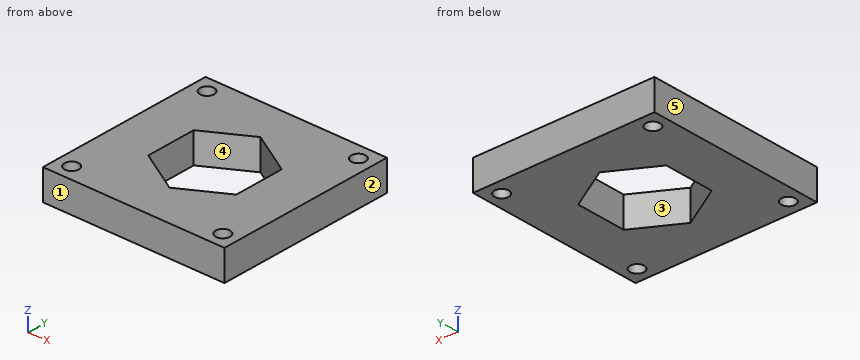
Autodesk Fusion 360 part; units mm, degrees
sketch "Sketch1" plane through (0, 0, 0) normal (0, 0, 1) x (1, 0, 0)
  line L0 (18.48, 10.6694) -> (0, 21.3389)
  line L1 (0, 21.3389) -> (-18.48, 10.6694)
  line L2 (-18.48, 10.6694) -> (-18.48, -10.6694)
  line L3 (-18.48, -10.6694) -> (0, -21.3389)
  line L4 (0, -21.3389) -> (18.48, -10.6694)
  line L5 (18.48, -10.6694) -> (18.48, 10.6694)
  line L6 (38.1, -38.1) -> (-38.1, -38.1)
  line L7 (-38.1, -38.1) -> (-38.1, 38.1)
  line L8 (-38.1, 38.1) -> (38.1, 38.1)
  line L9 (38.1, 38.1) -> (38.1, -38.1)
  line L10 (38.1, -38.1) -> (-38.1, 38.1) construction
  line L11 (-38.1, -38.1) -> (38.1, 38.1) construction
  line L12 (31.75, 31.75) -> (-31.75, 31.75) construction
  line L13 (-31.75, 31.75) -> (-31.75, -31.75) construction
  line L14 (-31.75, -31.75) -> (31.75, -31.75) construction
  line L15 (31.75, -31.75) -> (31.75, 31.75) construction
  line L16 (31.75, 31.75) -> (-31.75, -31.75) construction
  line L17 (-31.75, 31.75) -> (31.75, -31.75) construction
  circle A0 centre (-31.75, 31.75) radius 3
  circle A1 centre (-31.75, -31.75) radius 3
  circle A2 centre (31.75, -31.75) radius 3
  circle A3 centre (31.75, 31.75) radius 3
  dimension "d1" = 18.48
  dimension "d2" = 76.2
  dimension "d3" = 76.2
  dimension "d4" = 63.5
  dimension "d5" = 63.5
  dimension "d6" = 6
  dimension "d8" = 360
extrude "Extrude1" add sketch "Sketch1" along normal blind 12.7
sketch "Sketch2" plane through (0, 0, 12.7) normal (0, 0, 1) x (-1, 0, 0)
  circle A0 centre (31.75, 31.75) radius 3
  circle A1 centre (-31.75, -31.75) radius 3
  line L0 (-18.48, -10.6694) -> (-18.48, 10.6694)
  line L1 (-18.48, 10.6694) -> (0, 21.3389)
  line L2 (0, 21.3389) -> (18.48, 10.6694)
  line L3 (18.48, 10.6694) -> (18.48, -10.6694)
  line L4 (18.48, -10.6694) -> (0, -21.3389)
  line L5 (0, -21.3389) -> (-18.48, -10.6694)
  circle A2 centre (-31.75, 31.75) radius 3
  circle A3 centre (31.75, -31.75) radius 3
  line L6 (-38.1, -38.1) -> (38.1, -38.1)
  line L7 (38.1, -38.1) -> (38.1, 38.1)
  line L8 (38.1, 38.1) -> (-38.1, 38.1)
  line L9 (-38.1, 38.1) -> (-38.1, -38.1)
The listing builds one solid part. Answer for the finished solid, in the listing's coordinates (mm). Face numbers are marked on the shaded views. A direction names the side the tool comes from. Coordinates: 2 decimals unless noted, no trailing zeros. Write each loop counter-clockwise with the first axis right and the second up, starting at its lowest first coordinate (ties: lowest second). Pieces come first, ordered by that corner, then holes. Notation, with made-up numbers: M 17.5,16.25 L 53.5,16.25 A17 ccw 53.5,20.25 Z; hole C 24.5,-2.5 d1. An arc over 180 degrees is marked long. Put each result on its own line as item: value. Start each with the question number.
1. For a pull along Y with two mould halves and no side action, classify the marked faces 1, 2 and 3 as pulls with the +Y half, pulls with the -Y half, needs draft (parallel to the pull), parting line crosses it, or undercut.
2. A cutting plane is placed at A-A on z = 9.5. Write down the section's boundary in (x, y).
3. A cutting plane is placed at B-B on y = -31.75. Write down the section's boundary in (x, z), then the cut area to 3 significant figures.
4. A cutting plane is placed at C-C on x = 5. Write down the section's boundary in (y, z).
5. Consider line 1 (Y direction, x = 31.75, z = 6.75); line 2 (X direction, y = 31.5, z = 7.75); line 3 (X direction, y = -1.5, z = 4.5). Determine where each line is inside the solid, lowest interval first. Write a range as from..to.
6. Which of the six approach directions +Z, -Z, +X, -X, +Y, -Y give full straight-line access (tool end or side, diameter ignored) to the marked faces 4 and 5?
Resolved:
1. face 1: pulls with the -Y half
1. face 2: needs draft
1. face 3: undercut
2. outline: M -38.1,-38.1 L 38.1,-38.1 L 38.1,38.1 L -38.1,38.1 Z; hole C -31.75,-31.75 d6; hole C -31.75,31.75 d6; hole M -18.48,-10.67 L 0,-21.34 L 18.48,-10.67 L 18.48,10.67 L 0,21.34 L -18.48,10.67 Z; hole C 31.75,-31.75 d6; hole C 31.75,31.75 d6
3. outline: M -38.1,0 L -34.75,0 L -34.75,12.7 L -38.1,12.7 Z; M -28.75,0 L 28.75,0 L 28.75,12.7 L -28.75,12.7 Z; M 34.75,0 L 38.1,0 L 38.1,12.7 L 34.75,12.7 Z
3. area: 815 mm2
4. outline: M -38.1,0 L -18.45,0 L -18.45,12.7 L -38.1,12.7 Z; M 18.45,0 L 38.1,0 L 38.1,12.7 L 18.45,12.7 Z
5. line 1: y = -38.1..-34.75, -28.75..28.75, 34.75..38.1
5. line 2: x = -38.1..-34.74, -28.76..28.76, 34.74..38.1
5. line 3: x = -38.1..-18.48, 18.48..38.1
6. face 4: +Z, -Z
6. face 5: +Z, -Z, -X, +Y, -Y
